```python
from build123d import *

# Parameters (mm, degrees)
SKETCH1_W               = 279.4
SKETCH1_H               = 279.4
BOSS_EXTRUDE1_DEPTH     = 12.7
SKETCH2_W               = 25.4
SKETCH2_H               = 12.7
BOSS_EXTRUDE2_DEPTH     = 12.7
LPATTERN1_COUNT         = 5
LPATTERN1_PITCH         = 50.8
MIRROR1_COPY_1_SKETCH_W = 25.4
MIRROR1_COPY_1_SKETCH_H = 12.7
MIRROR1_COPY_1_DEPTH    = 12.7
MIRROR1_COPY_2_SKETCH_W = 25.4
MIRROR1_COPY_2_SKETCH_H = 12.7
MIRROR1_COPY_2_DEPTH    = 12.7
MIRROR1_COPY_3_SKETCH_W = 25.4
MIRROR1_COPY_3_SKETCH_H = 12.7
MIRROR1_COPY_3_DEPTH    = 12.7
MIRROR1_COPY_4_SKETCH_W = 25.4
MIRROR1_COPY_4_SKETCH_H = 12.7
MIRROR1_COPY_4_DEPTH    = 12.7
SKETCH3_W               = 25.4
SKETCH3_H               = 12.7
BOSS_EXTRUDE3_DEPTH     = 12.7
LPATTERN2_COUNT         = 5
LPATTERN2_PITCH         = 50.8
SKETCH6_R               = 4.7625
CUT_EXTRUDE1_DEPTH      = 13.7
SKETCH8_W               = 88.066093183
SKETCH8_H               = 177.8
CUT_EXTRUDE3_DEPTH      = 13.7
SKETCH9_W               = 25.4
SKETCH9_H               = 12.7
BOSS_EXTRUDE4_DEPTH     = 12.7


with BuildPart() as part:
    # Sketch1 → Boss-Extrude1 (new body)
    with BuildSketch(Plane(origin=(0, 0, 0), x_dir=(1, 0, 0), z_dir=(0, 1, 0))):
        Rectangle(SKETCH1_W, SKETCH1_H)
    extrude(amount=BOSS_EXTRUDE1_DEPTH)

    # Sketch2 → Boss-Extrude2 (add)
    with BuildSketch(Plane(origin=(139.7, 0, 0), x_dir=(0, 0, -1), z_dir=(1, 0, 0))):
        with Locations((-127, 6.35)):
            Rectangle(SKETCH2_W, SKETCH2_H)
    boss_extrude2 = extrude(amount=BOSS_EXTRUDE2_DEPTH)

    # LPattern1: Boss-Extrude2 ×5
    with Locations(*[(0, 0, -i * LPATTERN1_PITCH) for i in range(1, LPATTERN1_COUNT)]):
        add(boss_extrude2)

    # Mirror1: Boss-Extrude2 across plane
    add(boss_extrude2.mirror(Plane(origin=(0, 0, 0), x_dir=(0, 0, 1), z_dir=(1, 0, 0))))

    # Mirror1 copy 1 sketch → Mirror1 copy 1 (add)
    with BuildSketch(Plane(origin=(-139.7, 0, -50.8), x_dir=(0, 0, -1), z_dir=(-1, 0, 0))):
        with Locations((-127, -6.35)):
            Rectangle(MIRROR1_COPY_1_SKETCH_W, MIRROR1_COPY_1_SKETCH_H)
    extrude(amount=MIRROR1_COPY_1_DEPTH)

    # Mirror1 copy 2 sketch → Mirror1 copy 2 (add)
    with BuildSketch(Plane(origin=(-139.7, 0, -101.6), x_dir=(0, 0, -1), z_dir=(-1, 0, 0))):
        with Locations((-127, -6.35)):
            Rectangle(MIRROR1_COPY_2_SKETCH_W, MIRROR1_COPY_2_SKETCH_H)
    extrude(amount=MIRROR1_COPY_2_DEPTH)

    # Mirror1 copy 3 sketch → Mirror1 copy 3 (add)
    with BuildSketch(Plane(origin=(-139.7, 0, -152.4), x_dir=(0, 0, -1), z_dir=(-1, 0, 0))):
        with Locations((-127, -6.35)):
            Rectangle(MIRROR1_COPY_3_SKETCH_W, MIRROR1_COPY_3_SKETCH_H)
    extrude(amount=MIRROR1_COPY_3_DEPTH)

    # Mirror1 copy 4 sketch → Mirror1 copy 4 (add)
    with BuildSketch(Plane(origin=(-139.7, 0, -203.2), x_dir=(0, 0, -1), z_dir=(-1, 0, 0))):
        with Locations((-127, -6.35)):
            Rectangle(MIRROR1_COPY_4_SKETCH_W, MIRROR1_COPY_4_SKETCH_H)
    extrude(amount=MIRROR1_COPY_4_DEPTH)

    # Sketch3 → Boss-Extrude3 (add)
    with BuildSketch(Plane(origin=(0, 0, -139.7), x_dir=(-1, 0, 0), z_dir=(0, 0, -1))):
        with Locations((-101.6, 6.35)):
            Rectangle(SKETCH3_W, SKETCH3_H)
    boss_extrude3 = extrude(amount=BOSS_EXTRUDE3_DEPTH)

    # LPattern2: Boss-Extrude3 ×5
    with Locations(*[(-i * LPATTERN2_PITCH, 0, 0) for i in range(1, LPATTERN2_COUNT)]):
        add(boss_extrude3)

    # Sketch6 → Cut-Extrude1 (cut, through all)
    with BuildSketch(Plane(origin=(0, 12.7, 0), x_dir=(1, 0, 0), z_dir=(0, 1, 0))):
        with Locations((38.1, 11.176)):
            Circle(SKETCH6_R)
    extrude(amount=-CUT_EXTRUDE1_DEPTH, mode=Mode.SUBTRACT)

    # Sketch8 → Cut-Extrude3 (cut, through all)
    with BuildSketch(Plane(origin=(0, 12.7, 0), x_dir=(1, 0, 0), z_dir=(0, 1, 0))):
        with Locations((-108.366953408, 0)):
            Rectangle(SKETCH8_W, SKETCH8_H)
    extrude(amount=-CUT_EXTRUDE3_DEPTH, mode=Mode.SUBTRACT)

    # Sketch9 → Boss-Extrude4 (add)
    with BuildSketch(Plane.ZY.offset(139.7)):
        with Locations((-101.6, 6.35)):
            Rectangle(SKETCH9_W, SKETCH9_H)
    extrude(amount=BOSS_EXTRUDE4_DEPTH)


solid = part.part
```
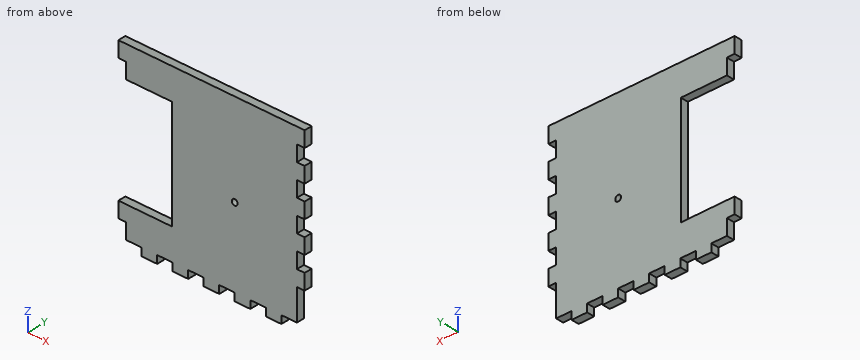
Part model, mm, in its own coordinate system. Round coordinates to 2 decimals unless told otherwise and drop trailing zeros. Loops run counter-clockwise (first coordinate to the right, second up) from the corner with the lowest first, then second, coordinate; pieces in that order, holes last.
Item 1: Drop flat-ended pins along their axis: P1, Ø4, axis at y = 8.5, z = -147, coming from the +X side; P2, Ø4, axis at y = 4, z = 60, coming from the +X side; P3, Ø5, axis at y = 3, z = 45, coming from the -X side. Give the stop position or say it passes through.
Item 2: Cut at B-B, the plane z = 51.5. Give the cut face in (x, y).
Item 3: Cut at C-C, the plane x = -23.5. Give the cut face in (y, z).
Item 4: Cut at A-A, the plane x = -109. Give the cut face in (y, z).
Item 5: Drill centre lines: line 1 (Z direction, x = -108, y = 8); line 2 (X direction, y = 1.5, z = -115); line 3 (X direction, y = 9.5, z = -33). Where is each one in solid material? Low to high.
A:
1. P1: stops at x = 114.3
1. P2: stops at x = 139.7
1. P3: stops at x = -64.33
2. outline: (-64.33, 0) - (139.7, 0) - (139.7, 12.7) - (-64.33, 12.7) - close
3. outline: (0, -139.7) - (12.7, -139.7) - (12.7, 139.7) - (0, 139.7) - close
4. outline: (0, -152.4) - (12.7, -152.4) - (12.7, -88.9) - (0, -88.9) - close; (0, 88.9) - (12.7, 88.9) - (12.7, 139.7) - (0, 139.7) - close
5. line 1: z = -152.4 to -88.9, 88.9 to 139.7
5. line 2: x = -139.7 to 139.7
5. line 3: x = -64.33 to 152.4
